```python
from build123d import *

# Parameters (mm, degrees)
SKETCH1_R           = 12.6
SKETCH1_R_2         = 6.55
BOSS_EXTRUDE1_DEPTH = 6.5
SKETCH2_R           = 1.095
CUT_EXTRUDE1_DEPTH  = 13.6
SKETCH4_R           = 12.6
SKETCH4_R_2         = 5.55
BOSS_EXTRUDE2_DEPTH = 1.82
CUT_EXTRUDE2_DEPTH  = 6.5
CIRPATTERN1_COUNT   = 3


with BuildPart() as part:
    # Sketch1 → Boss-Extrude1 (new body)
    with BuildSketch(Plane(origin=(0, 0, 0), x_dir=(1, 0, 0), z_dir=(0, 1, 0))):
        with Locations(Location((0, 0, 0), (0, 0, 270))):  # turned: the seam where the file's is
            Circle(SKETCH1_R)
        with Locations(Location((0, 0, 0), (0, 0, 270))):  # turned: the seam where the file's is
            Circle(SKETCH1_R_2, mode=Mode.SUBTRACT)
    extrude(amount=BOSS_EXTRUDE1_DEPTH)

    # Sketch2 → Cut-Extrude1 (cut, through all)
    with BuildSketch(Plane(origin=(0, 0, 0), x_dir=(0, 0, -1), z_dir=(1, 0, 0))):
        with Locations((0, 4.25)):
            Circle(SKETCH2_R)
    cut_extrude1 = extrude(amount=-CUT_EXTRUDE1_DEPTH, mode=Mode.SUBTRACT)

    # Sketch4 → Boss-Extrude2 (add)
    with BuildSketch(Plane.XZ):
        with Locations(Location((0, 0, 0), (0, 0, 270))):  # turned: the seam where the file's is
            Circle(SKETCH4_R)
        with Locations(Location((0, 0, 0), (0, 0, 270))):  # turned: the seam where the file's is
            Circle(SKETCH4_R_2, mode=Mode.SUBTRACT)
    extrude(amount=BOSS_EXTRUDE2_DEPTH)

    # Sketch3 → Cut-Extrude2 (cut)
    with BuildSketch(Plane(origin=(0, 6.5, 0), x_dir=(1, 0, 0), z_dir=(0, 1, 0))):
        with BuildLine():
            ThreePointArc((5.3628125, 3.760683726), (8, 0), (5.3628125, -3.760683726))
            ThreePointArc((5.3628125, -3.760683726), (6.55, 0), (5.3628125, 3.760683726))
        make_face()
    extrude(amount=-CUT_EXTRUDE2_DEPTH, mode=Mode.SUBTRACT)

    # CirPattern1: Cut-Extrude1 ×3 about axis
    cirpattern1_axis = Axis((0, 6.875, 0), (0, -1, 0))
    for i in range(1, CIRPATTERN1_COUNT):
        add(cut_extrude1.rotate(cirpattern1_axis, i * 360 / CIRPATTERN1_COUNT), mode=Mode.SUBTRACT)


solid = part.part
```
CAD build for the part. Positions are in the model's coordinates, mm. A direction names the side the tool comes from. Coordinates: 2 decimals unless noted, no trailing zeros. Order: outer loops, then holes, each group sorted by start corner. A loop starts at its lowest first (then second) coordinate and runs counter-clockwise, first axis right, second up. Notation, with made-up numbers: (56.5, 14.5) -> (110.5, 14.5) arc R18 ccw to (110.5, 36.5) -> close; hole circle Ø4 at (4.5, 47). An arc over 180 degrees is marked (long way). Use one line per item in the form item = value. Start each with the question number.
1) Band-saw the part on A-A on x = 0. Give the cut face in (y, z), then the cut area to 3 significant figures.
2) Drop flat-ended pins along their axis: pin 1 (4 mm diameter, centred on y = -1, z = 3.5, fed in from -X); pin 2 (13 mm diameter, centred on x = 0, z = 0, fed in from +Y); pin 3 (1.5 mm diameter, centred on y = -1, z = -5.5, fed in from +X). Give the stop position or say it passes through.
3) Band-saw the part on C-C on y = 4.25. Give the cut face in (x, z) (3 decimals), then the cut area to 3 significant figures.
4) Pull direction Y, two halves, no side cores. Call faces 4 (the flat face through (-3, -1.82, -5)), 5 (the cylindrical face through (4.95, 3.18, 8.1)), 6 (the cylindrical face through (8, 3, 0)), 7 (the flat face through (-5, 6.5, 5)): +Y half, -Y half, draft (parallel to the pull), parting line (faces both ways), or undercut.
5) Band-saw the part on D-D on x = -3.75. Give the cut face in (y, z), then the cut area to 3 significant figures.
6) Drill centre lines: L1, parallel to X at y = -0.5, z = 0; L2, parallel to Z at x = 0, y = 4; L3, parallel to X at y = 1.5, z = -4.25. Where is each one in solid material? Low to high. Write a range as [from, to].
7) Tool access for faces 1 (the cylindrical face through (-6.546, 2.482, -0.232)), 2 (the cylindrical face through (4.54, 3.18, -8.33)), 3 (the cylindrical face through (-9.48, 3.18, 0.24)): list every direction of +Z, -Z, +X, -X, +Y, -Y with a clear straight run to the whole face (end or side of a thin tool).
8) Band-saw the part on B-B on z = 0. Give the cut face in (x, y) (3 decimals), then the cut area to 3 significant figures.
Entries:
q1.outline = (-1.82, -12.6) -> (6.5, -12.6) -> (6.5, -6.55) -> (0, -6.55) -> (0, -5.55) -> (-1.82, -5.55) -> close; (-1.82, 5.55) -> (0, 5.55) -> (0, 6.55) -> (6.5, 6.55) -> (6.5, 12.6) -> (-1.82, 12.6) -> close
q1.area = 104 mm2
q2.pin_1 = -12.51
q2.pin_2 = 0
q2.pin_3 = 11.67
q3.outline = (-12.552, -1.095) arc R12.6 ccw to (5.328, -11.418) -> (2.281, -6.14) arc R6.55 cw to (-6.458, -1.095) -> close; (-12.552, 1.095) -> (-6.458, 1.095) arc R6.55 cw to (2.281, 6.14) -> (5.328, 11.418) arc R12.6 ccw to start; (4.177, -5.045) -> (7.224, -10.323) arc R12.6 ccw to (7.224, 10.323) -> (4.177, 5.045) arc R6.55 cw to (5.363, 3.761) arc R4 cw to (5.363, -3.761) arc R6.55 cw to start
q3.area = 316 mm2
q4.face_4 = -Y half
q4.face_5 = undercut
q4.face_6 = draft
q4.face_7 = +Y half
q5.outline = (-1.82, -12.03) -> (6.5, -12.03) -> (6.5, -5.37) -> (0, -5.37) -> (0, -4.09) -> (-1.82, -4.09) -> close; (-1.82, 4.09) -> (0, 4.09) -> (0, 5.37) -> (6.5, 5.37) -> (6.5, 12.03) -> (-1.82, 12.03) -> close
q5.area = 115 mm2
q6.L1 = [-12.6, -5.55], [5.55, 12.6]
q6.L2 = [-12.6, -6.55], [6.55, 12.6]
q6.L3 = [-11.86, -4.98], [4.98, 11.86]
q7.face_1 = +Y
q7.face_2 = none
q7.face_3 = -X
q8.outline = (-12.6, -1.82) -> (-5.55, -1.82) -> (-5.55, 0) -> (-6.55, 0) -> (-6.55, 3.155) -> (-12.6, 3.155) -> close; (-12.6, 5.345) -> (-6.55, 5.345) -> (-6.55, 6.5) -> (-12.6, 6.5) -> close; (5.55, -1.82) -> (12.6, -1.82) -> (12.6, 6.5) -> (8, 6.5) -> (8, 0) -> (5.55, 0) -> close
q8.area = 81.6 mm2
